Build history of the part. All positions in model axes, mm. Face numbers are marked on the shaded views. Round coordinates to 2 decimals unless told otherwise and drop trailing zeros. Loops run counter-clockwise (first coordinate to the right, second up) from the corner with the lowest first, then second, coordinate; pieces in that order, holes last.
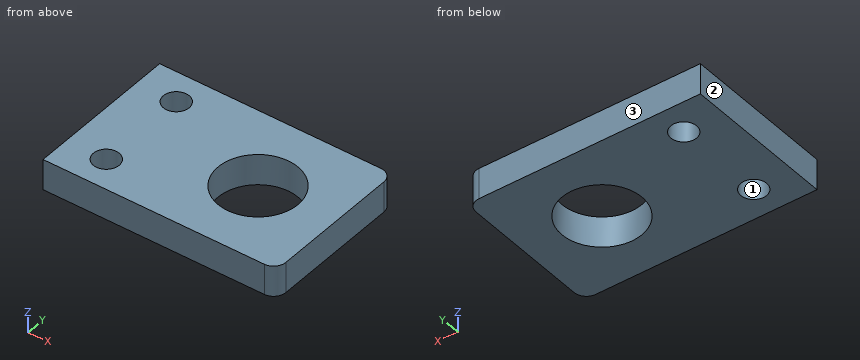
from build123d import *

# Parameters (mm, degrees)
SKETCH_1_R      = 2.1
SKETCH_1_R_2    = 6.5
EXTRUDE_1_DEPTH = 5


with BuildPart() as part:
    # 草图1 → 凸台-拉伸1 (new body)
    with BuildSketch(Plane.XY):
        with BuildLine():
            Line((-16.515544041, 16.418393782), (19.484455959, 16.418393782))
            ThreePointArc((19.484455959, 16.418393782), (20.898669521, 15.832607345), (21.484455959, 14.418393782))
            Line((21.484455959, 14.418393782), (21.484455959, -6.581606218))
            ThreePointArc((21.484455959, -6.581606218), (20.898669521, -7.99581978), (19.484455959, -8.581606218))
            Line((19.484455959, -8.581606218), (-16.515544041, -8.581606218))
            Line((-16.515544041, -8.581606218), (-16.515544041, 16.418393782))
        make_face()
        with Locations((-10.015544041, -3.581606218)):
            Circle(SKETCH_1_R, mode=Mode.SUBTRACT)
        with Locations((-10.015544041, 11.418393782)):
            Circle(SKETCH_1_R, mode=Mode.SUBTRACT)
        with Locations((8.984455959, 3.918393782)):
            Circle(SKETCH_1_R_2, mode=Mode.SUBTRACT)
    extrude(amount=EXTRUDE_1_DEPTH)


solid = part.part
(1) Slice it at B-B on x = 5.5. List the corners of the cut face in (y, z).
Responses:
outline: (-8.58, 0) - (-1.57, 0) - (-1.57, 5) - (-8.58, 5) - close; (9.41, 0) - (16.42, 0) - (16.42, 5) - (9.41, 5) - close
(2) Pull direction X, two halves, no side cores. Call the marked faces 1, 2 and 3: +X half, -X half, draft (parallel to the pull), parting line (faces both ways), or undercut.
Responses:
face 1: undercut
face 2: -X half
face 3: draft
(3) Slice it at C-C on z = 3. List the corners of the cut face in (x, y), plus the area to 3 significant figures.
Responses:
outline: (-16.52, -8.58) - (19.48, -8.58) arc R2 ccw to (21.48, -6.58) - (21.48, 14.42) arc R2 ccw to (19.48, 16.42) - (-16.52, 16.42) - close; hole circle Ø4.2 at (-10.02, -3.58); hole circle Ø4.2 at (-10.02, 11.42); hole circle Ø13 at (8.98, 3.92)
area: 788 mm2
(4) Slice it at A-A on y = 4.75. List the corners of the cut face in (x, z).
Responses:
outline: (-16.52, 0) - (2.54, 0) - (2.54, 5) - (-16.52, 5) - close; (15.43, 0) - (21.48, 0) - (21.48, 5) - (15.43, 5) - close
(5) Probe line 1 (Y direction, x = -10, z = 0.95); line 2 (X direction, y = 8.75, z = 4.15); line 3 (Y direction, x = 11, z = 2.8). List the from-to ranges inside material, lowest first.
Responses:
line 1: y = -8.58 to -5.68, -1.48 to 9.32, 13.52 to 16.42
line 2: x = -16.52 to 4.64, 13.33 to 21.48
line 3: y = -8.58 to -2.26, 10.1 to 16.42
